Can you work these out from the model? Positions are in its coordinate system, mm. A direction names the side the tool comes from. Give positions to 0.01 mm unless a question says otherwise; leave off trailing zeros. Loops run counter-clockwise (first coordinate to the right, second up) from the corner with the lowest first, then second, coordinate; pieces in that order, holes last. Notation, with made-up numbers: (16.5, 87) -> (66.5, 87) arc R15 ccw to (66.5, 104) -> close; hole circle Ø4 at (-15, 3.25). An arc over 180 degrees is marked (long way). One line per question, with ' | ' between items.
from build123d import *

# Parameters (mm, degrees)
SKETCH1_R          = 11.43413059
BASE_EXTRUDE_DEPTH = 40.360136162
DOME1_FACE_RADIUS  = 11.43413059
DOME1_HEIGHT       = 2.54
SKETCH2_OUTSIDE_W  = 35.612
SKETCH2_OUTSIDE_H  = 35.612
SKETCH2_OUTSIDE_R  = 8.14940086
CUT_EXTRUDE1_DEPTH = 18.034


with BuildPart() as part:
    # Sketch1 → Base-Extrude (new body)
    with BuildSketch(Plane.XY):
        with Locations((-45.925033829, 18.948035519)):
            Circle(SKETCH1_R)
    extrude(amount=BASE_EXTRUDE_DEPTH)

    # Dome1: an elliptical dome of height H over a round flat face of radius A is half a spheroid: the quarter ellipse of half axes A and H revolved about the face's axis
    with BuildSketch(Plane((-45.925033829, 18.948035519, 40.360136162), x_dir=(0, 1, 0), z_dir=(1, 0, 0)), mode=Mode.PRIVATE) as dome1_quarter:
        Ellipse(DOME1_FACE_RADIUS, DOME1_HEIGHT)
        Rectangle(DOME1_FACE_RADIUS, DOME1_HEIGHT, align=(Align.MIN, Align.MIN), mode=Mode.INTERSECT)
    revolve(dome1_quarter.sketch, axis=Axis((-45.925033829, 18.948035519, 40.360136162), (0, 0, 1)))

    # Sketch2 outside → Cut-Extrude1 (cut)
    with BuildSketch(Plane(origin=(0, 0, 0), x_dir=(-1, 0, 0), z_dir=(0, 0, -1))):
        with Locations((45.925, 18.948)):
            Rectangle(SKETCH2_OUTSIDE_W, SKETCH2_OUTSIDE_H)
        with Locations((45.925033829, 18.948035519)):
            Circle(SKETCH2_OUTSIDE_R, mode=Mode.SUBTRACT)
    extrude(amount=-CUT_EXTRUDE1_DEPTH, mode=Mode.SUBTRACT)


solid = part.part
Q1. If we section it at B-B (z = 33): Write out the boundary of the cut face in (x, y).
Entries:
outline: circle Ø22.87 at (-45.93, 18.95)
Q2. If we section it at A-A (z = 15): Write out the boundary of the cut face in (x, y).
Entries:
outline: circle Ø16.3 at (-45.93, 18.95)
Q3. On a 3-axis mill with a long thin cutter (end or side, diameter ignored), from which of +Z, -Z, +X, -X, +Y, -Y can I reach the whole of each face in a straight line? I mean faces 1 (the face through (-57.35, 19.45, 29.04)), 2 (the face through (-38, 22, 18.034)). Say none if no direction works.
Entries:
face 1: +Z, -Z | face 2: -Z
Q4. For pin 1 Ø2 at (x, y) = (-42, 18.5) entering from +Z; pin 2 Ø1 at (x, z) = (-49, 28.5) entering from -Y; pin 3 Ø8 at (y, z) = (10, 21) entering from -X, each with a flat end and sliding along its axis, tell me the tip position at first contact or that it passes through.
Entries:
pin 1: z = 42.81 | pin 2: y = 7.81 | pin 3: x = -56.23
Q5. If I drill on probe 1 along X at (y, z) = (19.25, 32); probe 2 along Y at (x, z) = (-50.25, 23); probe 3 along Z at (x, y) = (-55.5, 19), over which ranges is the centre line in solid material (lowest first)? Write a range as from..to.
Entries:
probe 1: -57.36..-34.49 | probe 2: 8.36..29.53 | probe 3: 18.03..41.75
